Could you check a few things on this model? Use its own coordinates, in mm. A direction names the side the tool comes from. Round coordinates to 2 decimals unless told otherwise and drop trailing zeros. Loops run counter-clockwise (first coordinate to the right, second up) from the corner with the lowest first, then second, coordinate; pieces in that order, holes last. Notation, with made-up numbers: (54, 8) - (94, 8) arc R10 ccw to (94, 16) - close; hole circle Ø6 at (25.5, 6). An arc over 180 degrees is marked (long way). Use one line per item in the form item = value.
Autodesk Inventor part; units mm, degrees
ref_plane "YZ Plane" through (0, 0, 0) normal (1, 0, 0) x (0, 1, 0)
ref_plane "XZ Plane" through (0, 0, 0) normal (0, 1, 0) x (-1, 0, 0)
ref_plane "XY Plane" through (0, 0, 0) normal (0, 0, 1) x (1, 0, 0)
sketch "Sketch1" plane through (0, 0, 0) normal (0, 0, 1) x (1, 0, 0)
  circle A0 centre (0, 0) radius 1.5
  circle A1 centre (0, 0) radius 5.5
  circle A2 centre (0, 0) radius 3.5
  dimension "d0" = 3
  dimension "d1" = 11
  dimension "d2" = 7
extrude "Extrusion1" add sketch "Sketch1" along normal mid plane 30 contours A1
extrude "Extrusion2" add sketch "Sketch1" along normal blind 15 contours A2
extrude "Extrusion3" add sketch "Sketch1" along normal mid plane 5 contours A0
extrude "Extrusion4" add sketch "Sketch1" against normal blind 2.5 contours A2
properties part number "Shaft Coupler"
1. We'd pull the mould along Y, two halves only. Please class faces 1 (the face through (-1.3, -1.1, 15)), 2 (the face through (-1.19, -5.37, 0.21)), 3 (the face through (0, 0, -2.5)), 4 (the face through (-1.5, -0.07, 8.66)): +Y half, -Y half, draft (parallel to the pull), parting line (faces both ways), or undercut.
Solution:
face_1 = draft
face_2 = parting line
face_3 = undercut
face_4 = undercut
2. On a 3-axis mill with a long thin cutter (end or side, diameter ignored), from which of +Z, -Z, +X, -X, +Y, -Y can I reach the whole of each face in a straight line? I mean faces 5 (the face through (3.233, -1.341, -8.662)), 6 (the face through (4, 0, -15)), 7 (the face through (0, 0, 2.5)). Say none if no direction works.
Solution:
face_5 = -Z
face_6 = -Z, +X, -X, +Y, -Y
face_7 = +Z
3. If we section it at A-A, the plane x = 0: Write out the boundary of the cut face in (y, z).
Solution:
outline = (-5.5, -15) - (-3.5, -15) - (-3.5, -2.5) - (3.5, -2.5) - (3.5, -15) - (5.5, -15) - (5.5, 15) - (1.5, 15) - (1.5, 2.5) - (-1.5, 2.5) - (-1.5, 15) - (-5.5, 15) - close
4. For P1, Ø3.5, axis at x = 1, y = 1, coming from the -Z side; P2, Ø2, axis at x = 2, z = 4, coming from the +Y side; P3, Ø1.5, axis at x = 0, y = -0.5, coming from the +Z side, each with a flat end and sliding along its axis, tell me the tip position at first contact or that it passes through.
Solution:
P1 = -2.5
P2 = 5.41
P3 = 2.5
5. If we section it at D-D, the plane y = 2.5: Write out the boundary of the cut face in (x, z), plus the area to 3 significant figures.
Solution:
outline = (-4.9, -15) - (-2.45, -15) - (-2.45, -2.5) - (2.45, -2.5) - (2.45, -15) - (4.9, -15) - (4.9, 15) - (-4.9, 15) - close
area = 233 mm^2
6. Please list where these lines run through material, in increasing order: line 1 along Y through (x, z) = (0, -10.5); line 2 along Y through (x, z) = (0, 7); line 3 along X through (y, z) = (-2, -3.75).
Solution:
line_1 = -5.5 to -3.5, 3.5 to 5.5
line_2 = -5.5 to -1.5, 1.5 to 5.5
line_3 = -5.12 to -2.87, 2.87 to 5.12
7. If we section it at B-B, the plane z = -3.75: Write out the boundary of the cut face in (x, y).
Solution:
outline = circle Ø11 at (0, 0); hole circle Ø7 at (0, 0)
